Geometry: final body of the model. Coordinates: model frame, mm. Give positions to 0.01 mm unless a question says otherwise; leave off trailing zeros. Write each loop counter-clockwise with the first axis right and the second up, starting at its lowest first coordinate (ties: lowest second). Pieces come first, ordered by that corner, then holes. Notation, with made-up numbers: M -15,-9 L 3,-9 A28 ccw 3,17 Z; hole C -18.5,81 d6. An arc over 180 degrees is marked long. Use a Markdown table: item, result. Add a question column.
1) Pin query (flat end, axial travel): pin 1 (12 mm diameter, centred on x = 1, y = -7, fed in from -Z); pin 2 (2 mm diameter, centred on x = -65.5, y = -40.5, fed in from +Z); pin 3 (4 mm diameter, centred on x = -27, y = -37.5, fed in from -Z). Return the tip coordinate at first contact, or that it passes through.
2) Draft query along X for faces 1 (the cylindrical face through (27.13, -19.72, 66.34)), 2 (the flat face through (-96.401, -23, 24)), 3 (the cylindrical face through (-42.72, -19.72, 66.34)), 4 (the flat face through (65, -60.96, 52)). Return one class per face: +X half, -X half, draft (parallel to the pull), parting line (faces both ways), or undercut.
3) Section D-D on y = -33. Return the cut outline in (x, z), then the cut area to 3 significant figures.
4) Section B-B on y = -46.5. Return the cut outline in (x, z), then the cut area to 3 significant figures.
5) Line query: line 1 (Y direction, x = -8, z = 21); line 2 (Y direction, x = -86.5, z = -1.5); line 3 (X direction, y = -29.5, z = 23.5). Output: solid intervals per line, ascending.
6) Section C-C on z = 70. Return the cut outline in (x, y).
```python
from build123d import *

# Parameters (mm, degrees)
F1_DEPTH    = 60.96
F2_T2_ANGLE = 359.64
F3_SIZE     = 10.15999
F4_R        = 6.35
F5_DEPTH    = 25.4
F6_SIZE     = 1.27
F7_SIZE     = 5.08
F8_SIZE     = 5.08


# Not quite as in the source:
# - a fillet or chamfer that OpenCascade refuses, or shapes differently, is made with other operations: its cross-section is extruded or revolved along the edge and cut away or added
# - a fillet or chamfer is up to 0.001 mm smaller than in the source, because OpenCascade refuses the exact size


with BuildPart() as f1:
    # F0 (on Front) → F1 (new body)
    with BuildSketch(Plane.XZ):
        with BuildLine():
            Line((68.6990445861, 54.4476021031), (0, 54.4476021031))
            Line((0, 54.4476021031), (-96.4009554139, 54.4476021031))
            Line((-96.4009554139, 54.4476021031), (-96.4009554139, -24.6122339721))
            ThreePointArc((-96.4009554139, -24.6122339721), (-13.8509554139, 20.7245603096), (68.6990445861, -24.6122339721))
            Line((68.6990445861, -24.6122339721), (68.6990445861, 54.4476021031))
        make_face()
    extrude(amount=F1_DEPTH)

    # F2: chamfer of 50.8 on 1 edges, made by hand

    # F2_s1 → F2_t2 (revolve, cut)
    with BuildSketch(Plane(origin=(-13.6086096269, 0, 0.0427528487), x_dir=(0, 1, 0), z_dir=(0.9999950652, 0, -0.0031415875))):
        Polygon((-60.96, -225.7638003707), (-10.16, -174.9638003707), (-60.96, -174.9638003707), align=None)
    revolve(axis=Axis((-13.8509554139, -60.96, -77.0980532681), (0, 1, 0)), revolution_arc=F2_T2_ANGLE, mode=Mode.SUBTRACT)

    # F3 (size 10.16 in the source; OpenCascade refuses exactly that, so slightly less here)
    f3_edges = [f1.edges().sort_by_distance(p)[0] for p in [
        (-13.850955, -10.16, 20.72456),
    ]]
    chamfer(f3_edges, length=F3_SIZE)

    # F4 (on face) → F5 (join)
    with BuildSketch(Plane.XY.offset(54.4476021031)):
        with Locations((-48.7759554139, -21.6264873743)):
            Circle(F4_R)
        with Locations((21.0740445861, -21.6264873743)):
            Circle(F4_R)
    extrude(amount=F5_DEPTH)

    # F6
    f6_edges = [f1.edges().sort_by_distance(p)[0] for p in [
        (-55.125955, -21.626487, 79.847602),
        (14.724045, -21.626487, 79.847602),
    ]]
    chamfer(f6_edges, length=F6_SIZE)

    # F7
    f7_edges = [f1.edges().sort_by_distance(p)[0] for p in [
        (-13.850955, -17.344239, 27.9088),
    ]]
    chamfer(f7_edges, length=F7_SIZE)

    # F8
    f8_edges = [f1.edges().sort_by_distance(p)[0] for p in [
        (-13.850955, -20.936342, 31.500902),
    ]]
    chamfer(f8_edges, length=F8_SIZE)


solid = f1.part
```
Found:
| question | item | result |
|---|---|---|
| 1 | pin 1 | z = 19.82 |
| 1 | pin 2 | z = 54.45 |
| 1 | pin 3 | z = 45.35 |
| 2 | face 1 | undercut |
| 2 | face 2 | -X half |
| 2 | face 3 | undercut |
| 2 | face 4 | draft |
| 3 | outline | M -96.4,10.91 A120.66 cw 68.7,10.91 L 68.7,54.45 L -96.4,54.45 Z |
| 3 | area | 3,480 mm² |
| 4 | outline | M -96.4,28.66 A134.16 cw -40.22,54.45 L -96.4,54.45 Z; M 12.52,54.45 A134.16 cw 68.7,28.66 L 68.7,54.45 Z |
| 4 | area | 1,150 mm² |
| 5 | line 1 | -1.09 to 0 |
| 5 | line 2 | -15.32 to 0 |
| 5 | line 3 | -96.4 to -73.91, 46.21 to 68.7 |
| 6 | outline | C -48.78,-21.63 d12.7; C 21.07,-21.63 d12.7 |
